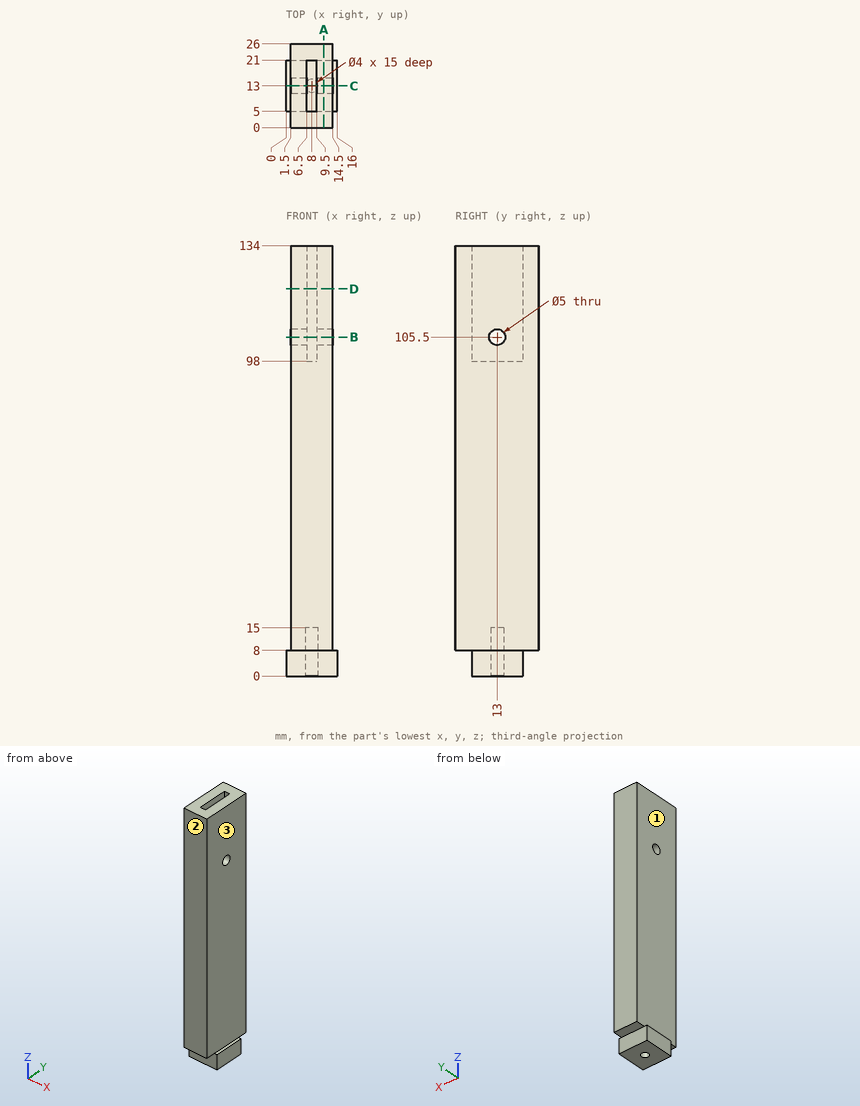
Verification items for this drawing (mm, ordinates from the low corner). A direction names the side the tool comes from. Coordinates: 2 decimals unless noted, no trailing zeros. Write each loop counter-clockwise with the first axis right and the second up, starting at its lowest first coordinate (ties: lowest second). Pieces come first, ordered by that corner, then holes. Notation, with made-up numbers: M 40,5.25 L 58,5.25 A17 cw 58,29.25 Z; hole C 1.25,80 d1. An arc over 180 degrees is marked long. Answer as a JSON object with one key per item and string values.
1. Section check C-C, the plane y = 13. Enter the section's corners in (x, z).
Answers below:
{"outline": "M 0,0 L 6,0 L 6,15 L 10,15 L 10,0 L 16,0 L 16,8 L 14.5,8 L 14.5,103 L 9.5,103 L 9.5,98 L 6.5,98 L 6.5,103 L 1.5,103 L 1.5,8 L 0,8 Z; M 1.5,108 L 6.5,108 L 6.5,134 L 1.5,134 Z; M 9.5,108 L 14.5,108 L 14.5,134 L 9.5,134 Z"}
2. Tool access check on the marked faces 1, 2 and 3. Record the directions out of +Z, -Z, +X, -X, +Y, -Y that give a thin tool (end or side, any length) a straight path to the whole face; none if there is none.
Answers below:
{"face 1": "+Z, -X, +Y, -Y", "face 2": "+Z, -Z, +X, -X, -Y", "face 3": "+Z, +X, +Y, -Y"}
3. Section check A-A, the plane x = 11.75. Enter the section's corners in (y, z), plus the area to 3 significant figures.
Answers below:
{"outline": "M 0,8 L 5,8 L 5,0 L 21,0 L 21,8 L 26,8 L 26,134 L 0,134 Z; hole C 13,105.5 d5", "area": "3,380 mm²"}
4. Section check D-D, the plane z = 120.5. Enter the section's corners in (x, y).
Answers below:
{"outline": "M 1.5,0 L 14.5,0 L 14.5,26 L 1.5,26 Z; hole M 6.5,5 L 9.5,5 L 9.5,21 L 6.5,21 Z"}
5. Go/stop test with flat-tipped pins: pin 1 Ø1.5 at (x, y) = (8.5, 16) entering from +Z; pin 2 Ø4 at (y, z) = (14.5, 103.5) entering from -X; pin 3 Ø3 at (x, y) = (8, 13) entering from -Z. Record where each tip stops, or that it passes through.
Answers below:
{"pin 1": "stops at z = 98", "pin 2": "stops at x = 1.5", "pin 3": "stops at z = 15"}
6. Section check B-B, the plane z = 105.5. Enter the section's corners in (x, y).
Answers below:
{"outline": "M 1.5,0 L 14.5,0 L 14.5,10.5 L 9.5,10.5 L 9.5,5 L 6.5,5 L 6.5,10.5 L 1.5,10.5 Z; M 1.5,15.5 L 6.5,15.5 L 6.5,21 L 9.5,21 L 9.5,15.5 L 14.5,15.5 L 14.5,26 L 1.5,26 Z"}
7. Scan lines: L1, parallel to Y at x = 8, z = 11; L2, parallel to Z at x = 13.2, y = 13; L3, parallel to Y at x = 11.55, z = 105.5. Record each from-to range of solid material in increasing order.
Answers below:
{"L1": "y = 0 to 11, 15 to 26", "L2": "z = 0 to 103, 108 to 134", "L3": "y = 0 to 10.5, 15.5 to 26"}
